Can you work these out from the model? Positions are in its coordinate system, mm. Face numbers are marked on the shaded views. A direction names the side the tool comes from. Give positions to 0.01 mm unless a question says otherwise; leave off trailing zeros. Order: outer loops, then holes, each group sorted by start corner. A loop starts at its lowest first (then second) coordinate and runs counter-clockwise, first axis right, second up.
Item 1: I'm going to push flat-ended pins straight in: pin 1 Ø8 at (x, z) = (56, -5) entering from +Y; pin 2 Ø12 at (x, y) = (68, 102.5) entering from -Z; pin 3 Ø0.8 at (y, z) = (43, -4) entering from -X (3 decimals). Where does each tip first touch, or does it pass through?
Item 2: I want a section at A-A, the plane x = 16. Write out the boundary of the cut face in (y, z).
Item 3: Which directions (+Z, -Z, +X, -X, +Y, -Y) give clear straight access to the entire face, cutting with the end or side of a thin tool? Please do the marked faces 3 and 4.
Item 4: I want a section at C-C, the plane z = -5. Write out the boundary of the cut face in (x, y) (3 decimals).
Item 5: If we mould it in two halves opening along X, with no side actions, what happens to the marked faces 1 and 2? For each: +X half, -X half, draft (parallel to the pull), parting line (faces both ways), or undercut.
Item 6: If I drill on line 1 along X through (y, z) = (156.5, 2.25) (3 decimals); line 2 along Y through (x, z) = (38.5, 1.25); line 3 along Z through (x, y) = (28, 140.5), over which ranges is the centre line in solid material (lowest first)?
Item 7: I want a section at B-B, the plane y = 75. Write out the boundary of the cut face in (x, z) (3 decimals).
Autodesk Inventor part; units mm, degrees
ref_plane "Płaszczyzna konstrukcyjna1" through (20.925, 15, -12) normal (0, 0, -1) x (0, 1, 0)
ref_plane "YZ Plane" through (0, 0, 0) normal (1, 0, 0) x (0, 1, 0)
ref_plane "XZ Plane" through (0, 0, 0) normal (0, 1, 0) x (-1, 0, 0)
sketch "Szkic1" plane through (0, 0, 0) normal (0, 0, 1) x (1, 0, 0)
  line L0 (12.425, 226.5) -> (77.425, 226.5)
  line L1 (77.425, 226.5) -> (77.425, 42.5)
  line L2 (77.425, 42.5) -> (12.425, 42.5)
  line L3 (12.425, 42.5) -> (12.425, 226.5)
extrude "Wyciągnięcie proste1" add sketch "Szkic1" along normal blind 4
shell "Skorupa1" thickness 1.5 removed faces 1 at (55.7583, 103.8333, 0)
ref_plane "Płaszczyzna konstrukcyjna1" through (20.925, 15, -12) normal (0, 0, -1) x (0, 1, 0)
sketch "Szkic2" plane through (0, 0, 0) normal (0, 0, -1) x (-1, 0, 0)
  line L0 (-13.925, 44) -> (-75.925, 44)
  line L1 (-77.425, 42.5) -> (-12.425, 42.5)
  line L2 (-22.425, 17.5) -> (-22.425, 215.5)
  arc A0 (-23.425, 16.5) -> (-22.425, 17.5) centre (-23.425, 17.5) ccw
  line L3 (-66.425, 16.5) -> (-23.425, 16.5)
  arc A1 (-67.425, 17.5) -> (-66.425, 16.5) centre (-66.425, 17.5) ccw
  line L4 (-67.425, 215.5) -> (-67.425, 17.5)
  arc A2 (-66.425, 216.5) -> (-67.425, 215.5) centre (-66.425, 215.5) ccw
  line L5 (-23.425, 216.5) -> (-66.425, 216.5)
  arc A3 (-22.425, 215.5) -> (-23.425, 216.5) centre (-23.425, 215.5) ccw
  line L6 (-20.925, 218) -> (-20.925, 15)
  line L7 (-68.925, 218) -> (-20.925, 218)
  line L8 (-68.925, 15) -> (-68.925, 218)
  line L9 (-20.925, 15) -> (-68.925, 15)
  line L10 (-1.5, 236.5) -> (-88.35, 236.5)
  line L11 (-88.35, 0) -> (-88.35, 236.5)
  line L12 (-88.35, 0) -> (-1.5, 0)
  line L13 (-1.5, 0) -> (-1.5, 236.5)
  line L14 (-68.925, 15) -> (-68.925, 218)
  line L15 (-68.925, 218) -> (-20.925, 218)
  line L16 (-20.925, 218) -> (-20.925, 15)
  line L17 (-20.925, 15) -> (-68.925, 15)
  line L18 (-22.425, 17.5) -> (-22.425, 215.5)
  arc A4 (-23.425, 16.5) -> (-22.425, 17.5) centre (-23.425, 17.5) ccw
  line L19 (-66.425, 16.5) -> (-23.425, 16.5)
  arc A5 (-67.425, 17.5) -> (-66.425, 16.5) centre (-66.425, 17.5) ccw
  line L20 (-67.425, 215.5) -> (-67.425, 17.5)
  arc A6 (-66.425, 216.5) -> (-67.425, 215.5) centre (-66.425, 215.5) ccw
  line L21 (-23.425, 216.5) -> (-66.425, 216.5)
  arc A7 (-22.425, 215.5) -> (-23.425, 216.5) centre (-23.425, 215.5) ccw
  line L22 (-20.925, 218) -> (-20.925, 15)
  line L23 (-68.925, 218) -> (-20.925, 218)
  line L24 (-68.925, 15) -> (-68.925, 218)
  line L25 (-20.925, 15) -> (-68.925, 15)
  line L26 (-68.925, 15) -> (-68.925, 218)
  line L27 (-1.5, 236.5) -> (-88.35, 236.5)
  line L28 (-88.35, 0) -> (-88.35, 236.5)
  line L29 (-88.35, 0) -> (-1.5, 0)
  line L30 (-1.5, 0) -> (-1.5, 236.5)
  line L31 (-68.925, 15) -> (-68.925, 218)
  line L32 (-68.925, 218) -> (-20.925, 218)
  line L33 (-20.925, 218) -> (-20.925, 15)
  line L34 (-20.925, 15) -> (-68.925, 15)
  line L35 (-67.425, 44) -> (-22.425, 44)
  line L36 (-22.425, 44) -> (-22.425, 42.5)
  line L37 (-22.425, 42.5) -> (-67.425, 42.5)
  line L38 (-67.425, 42.5) -> (-67.425, 44)
  point P0 (0, 0)
extrude "Wyciągnięcie proste2" add sketch "Szkic2" along normal up to surface (12 mm away) contours L2 L1 L4 L0
properties part number "TYLNA CZARNA OBUDOWA STOJAKA" material "Tworzywo sztuczne, nieprzezroczyste czarne"
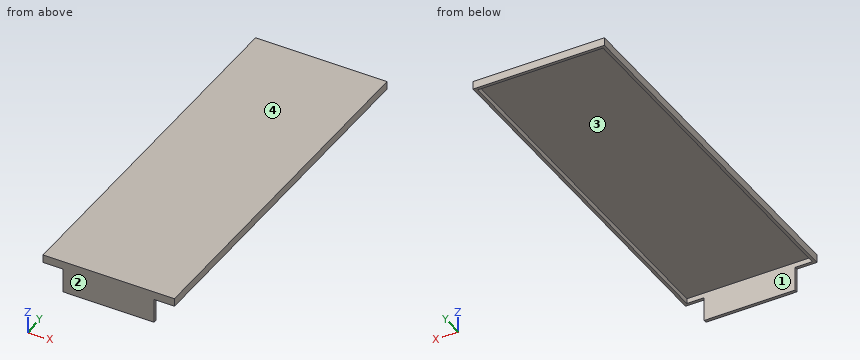
Results list:
1. pin 1: stops at y = 44
1. pin 2: stops at z = 2.5
1. pin 3: stops at x = 22.425
2. outline: (42.5, 0) - (44, 0) - (44, 2.5) - (225, 2.5) - (225, 0) - (226.5, 0) - (226.5, 4) - (42.5, 4) - close
3. face 3: -Z
3. face 4: +Z, +X, -X, +Y, -Y
4. outline: (22.425, 42.5) - (67.425, 42.5) - (67.425, 44) - (22.425, 44) - close
5. face 1: undercut
5. face 2: draft
6. line 1: x = 12.425 to 13.925, 75.925 to 77.425
6. line 2: y = 42.5 to 44, 225 to 226.5
6. line 3: z = 2.5 to 4
7. outline: (12.425, 0) - (13.925, 0) - (13.925, 2.5) - (75.925, 2.5) - (75.925, 0) - (77.425, 0) - (77.425, 4) - (12.425, 4) - close
